Input: part model. Units: mm. Frame: model coordinates. Coordinates: 2 decimals unless noted, no trailing zeros. Write each loop counter-clockwise with the first axis right and the second up, starting at its lowest first coordinate (ties: lowest second). Pieces come first, ordered by that corner, then holes. Notation, with made-up numbers: (77.25, 32) - (111.25, 32) arc R8 ccw to (111.25, 44) - close; hole circle Ø8 at (18.5, -14.5). An arc over 180 degrees is marked (long way). Put each result on its own line as item: value. Start each with the question number.
1. Cut plane A-A, the plane x = 0. Return loops of the section in (y, z), and give its area (3 significant figures).
2. Pull-direction query (Z, two-part tool) for faces 1 (the flat face through (0, 10, -2)), 2 (the cylindrical face through (-1.5, 4.93, -0.07)), 3 (the flat face through (-2.001, 4.93, 1.134)), 4 (the flat face through (0, 5, -2.3)); classes: released by +Z, released by -Z, zero draft, split by the parting line, or undercut.
3. Cut plane B-B, the plane y = 4.75. Return loops of the section in (x, z).
4. Cut plane D-D, the plane z = -2. Return loops of the section in (x, y).
5. Line query: line 1 (Z direction, x = 0, y = 2.5); line 2 (X direction, y = 8.75, z = 0.1); line 3 (X direction, y = 6, z = -0.85). Output: solid intervals per line, ascending.
6. Cut plane C-C, the plane z = -0.85. Return loops of the section in (x, y), and give its area (3 significant figures).
from build123d import *

# Parameters (mm, degrees)
SKETCH_1_R          = 1.5
EXTRUDE_2_DEPTH     = 5
SKETCH1_R           = 1.5
BOSS_EXTRUDE1_DEPTH = 5


with BuildPart() as part:
    # 草图1 → 凸台-拉伸2 (new body)
    with BuildSketch(Plane(origin=(0, 0, 0), x_dir=(1, 0, 0), z_dir=(0, 1, 0))):
        Polygon((-1.327905619, 2.3), (-2.655811238, 0), (-1.327905619, -2.3), (1.327905619, -2.3), (2.655811238, 0), (1.327905619, 2.3), align=None)
        Circle(SKETCH_1_R, mode=Mode.SUBTRACT)
    extrude(amount=EXTRUDE_2_DEPTH)

    # Sketch1 → Boss-Extrude1 (add)
    with BuildSketch(Plane(origin=(0, 5, 0), x_dir=(1, 0, 0), z_dir=(0, 1, 0))):
        Polygon((1.327905619, 2.3), (-1.327905619, 2.3), (-2.655811238, 0), (-1.327905619, -2.3), (1.327905619, -2.3), (2.655811238, 0), align=None)
        Circle(SKETCH1_R, mode=Mode.SUBTRACT)
    extrude(amount=BOSS_EXTRUDE1_DEPTH)


solid = part.part
Report:
1. outline: (0, -2.3) - (10, -2.3) - (10, -1.5) - (0, -1.5) - close; (0, 1.5) - (10, 1.5) - (10, 2.3) - (0, 2.3) - close
1. area: 16.0 mm^2
2. face 1: zero draft
2. face 2: undercut
2. face 3: released by +Z
2. face 4: released by -Z
3. outline: (-2.66, 0) - (-1.33, -2.3) - (1.33, -2.3) - (2.66, 0) - (1.33, 2.3) - (-1.33, 2.3) - close; hole circle Ø3 at (0, 0)
4. outline: (-1.5, 0) - (1.5, 0) - (1.5, 10) - (-1.5, 10) - close
5. line 1: z = -2.3 to -1.5, 1.5 to 2.3
5. line 2: x = -2.6 to -1.5, 1.5 to 2.6
5. line 3: x = -2.17 to -1.24, 1.24 to 2.17
6. outline: (-2.17, 0) - (-1.24, 0) - (-1.24, 10) - (-2.17, 10) - close; (1.24, 0) - (2.17, 0) - (2.17, 10) - (1.24, 10) - close
6. area: 18.6 mm^2
